Autodesk Inventor part; units mm, degrees
ref_plane "YZ Plane" through (0, 0, 0) normal (1, 0, 0) x (0, 1, 0)
ref_plane "XZ Plane" through (0, 0, 0) normal (0, 1, 0) x (-1, 0, 0)
ref_plane "XY Plane" through (0, 0, 0) normal (0, 0, 1) x (1, 0, 0)
sketch "Эскиз2" plane through (0, 0, 0) normal (1, 0, 0) x (0, 1, 0)
  line L0 (-30, 31) -> (-30, 23)
  line L1 (-30, 23) -> (-34, 23)
  line L2 (-34, 23) -> (-34, 11)
  line L3 (-34, 11) -> (-30, 11)
  line L4 (-30, 11) -> (-30, 0)
  line L5 (-30, 0) -> (-22, 0)
  line L6 (-22, 0) -> (-22, 4)
  line L7 (-22, 4) -> (-8, 4)
  line L8 (-8, 4) -> (-8, 0)
  line L9 (-8, 0) -> (0, 0)
  line L10 (0, 0) -> (0, 31) construction
  line L11 (30, 23) -> (34, 23)
  line L12 (34, 23) -> (34, 11)
  line L13 (34, 11) -> (30, 11)
  line L14 (30, 11) -> (30, 0)
  line L15 (30, 0) -> (22, 0)
  line L16 (22, 0) -> (22, 4)
  line L17 (22, 4) -> (8, 4)
  line L18 (8, 4) -> (8, 0)
  line L19 (8, 0) -> (0, 0)
  line L20 (-20, 7) -> (2, 7)
  line L21 (2, 7) -> (2, 11)
  line L22 (2, 11) -> (-20, 11)
  line L23 (-20, 11) -> (-20, 7)
  line L24 (-30, 31) -> (12, 31)
  line L25 (12, 31) -> (12, 21)
  line L26 (12, 21) -> (16, 21)
  line L27 (16, 21) -> (16, 27)
  line L28 (16, 27) -> (30, 27)
  line L29 (30, 27) -> (30, 23)
  point P0 (0, 0)
  dimension "d0" = 4
  dimension "d1" = 12
  dimension "d2" = 8
  dimension "d4" = 11
  dimension "d5" = 60
  dimension "d6" = 14
  dimension "d7" = 16
  dimension "d8" = 10
  dimension "d9" = 22
  dimension "d10" = 7
  dimension "d13" = 42
  dimension "d15" = 10
  dimension "d16" = 4
extrude "Выдавливание1" add sketch "Эскиз2" along normal blind 4
sketch "Эскиз3" plane through (4, 0, 0) normal (1, 0, 0) x (0, 0, -1)
  circle A0 centre (-11, 21) radius 1.5
  line L0 (-27, 30) -> (-27, 16)
  line L1 (0, 30) -> (-11, 30)
  point P0 (0, 0)
  dimension "d17" = 16
  dimension "d18" = 9
  dimension "d19" = 3
extrude "Выдавливание2" cut sketch "Эскиз3" against normal through all
properties part number "batBack" material "Дерево (береза)"
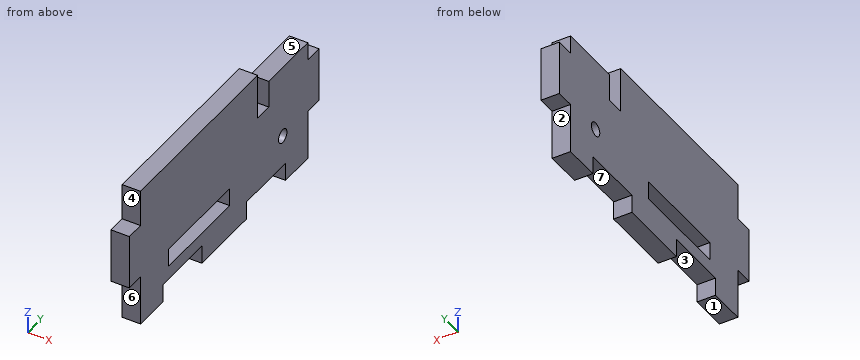
Work out the finished part from the listing and answer in its coordinate system (mm). Face numbers are marked on the shaded views. A direction names the side the tool comes from. Give positions to 0.01 mm unless a question says otherwise; leave off trailing zeros. Loops run counter-clockwise (first coordinate to the right, second up) from the corner with the lowest first, then second, coordinate; pieces in that order, holes last. Notation, with made-up numbers: (20, 46) -> (46, 46) arc R26 ccw to (46, 76) -> close; hole circle Ø9 at (59.25, 13). An arc over 180 degrees is marked (long way). Write item = value, one per line. Start each with the question number.
(1) Find section A-A on z = 24. Give the vertices of the cut face in (x, y).
(2) Find the intervals of material crossed by probe 1 along Y at (x, z) = (0.25, 3.5); probe 2 along Z at (x, y) = (0.3, -3.5); probe 3 along Z at (x, y) = (3.75, -14.5), in increasing order. Write a range as from..to.
(3) Find section B-B on y = 21. Give the vertices of the cut face in (x, z), and give its area (3 significant figures).
(4) Find section C-C on x = 1. Give the number of separate pieces and of enclosed holes in the cut face, and give its area (3 significant figures).
(5) Which of the six approach directions +Z, -Z, +X, -X, +Y, -Y give full straight-line access (tool end or side, diameter ignored) to the marked faces 4, 5, 6 and 7?
(6) Find section D-D on z = 28. Give the vertices of the cut face in (x, y), and give its area (3 significant figures).
(7) Given pin 1 Ø2 at (x, y) = (2, -16.5) entering from -Z; pin 2 Ø1.2 at (x, y) = (2, -31.5) entering from +Z; pin 3 Ø2 at (x, z) = (2, 1.5) entering from -Y, each flat-ended and moving along its own axis, determine where each tip first touches the part or whether it passes through.
(8) The mould has two halves that part along Y. Classify the marked faces 1, 2 and 3: +Y half, -Y half, draft (parallel to the pull), parting line (faces both ways), or undercut.
From the geometry:
q1.outline = (0, -30) -> (4, -30) -> (4, 12) -> (0, 12) -> close; (0, 16) -> (4, 16) -> (4, 30) -> (0, 30) -> close
q2.probe_1 = -30..-22, -8..8, 22..30
q2.probe_2 = 0..7, 11..31
q2.probe_3 = 4..7, 11..31
q3.outline = (0, 4) -> (4, 4) -> (4, 9.5) -> (0, 9.5) -> close; (0, 12.5) -> (4, 12.5) -> (4, 27) -> (0, 27) -> close
q3.area = 80.0 mm^2
q4.separate_pieces = 1
q4.enclosed_holes = 2
q4.area = 1,650 mm^2
q5.face_4 = +Z, +X, -X, -Y
q5.face_5 = +Z, +X, -X, +Y
q5.face_6 = -Z, +X, -X, -Y
q5.face_7 = -Z, +X, -X
q6.outline = (0, -30) -> (4, -30) -> (4, 12) -> (0, 12) -> close
q6.area = 168 mm^2
q7.pin_1 = 4
q7.pin_2 = 23
q7.pin_3 = -30
q8.face_1 = draft
q8.face_2 = +Y half
q8.face_3 = undercut
